Design review of the part built by this model. Coordinates are the model's own, in mm. A direction names the side the tool comes from. Give positions to 0.01 mm unless a question says otherwise; leave off trailing zeros. Write each loop counter-clockwise with the first axis right and the second up, starting at its lowest first coordinate (ties: lowest second). Pieces come first, ordered by that corner, then holes. Notation, with made-up numbers: (49.5, 36) -> (100.5, 36) arc R16 cw to (100.5, 57) -> close; hole circle Ø9 at (-23.75, 46). An arc over 180 degrees is marked (long way). Put each result on its own line as item: value. Start each with the question number.
from build123d import *

# Parameters (mm, degrees)
SCHIZZO4_R               = 2
TAGLIO_ESTRUSIONE1_DEPTH = 8


with BuildPart() as part:
    # Schizzo3 → Rivoluzione1 (revolve)
    with BuildSketch(Plane(origin=(0, 0, 0), x_dir=(1, 0, 0), z_dir=(0, 1, 0))):
        Polygon((0, 0), (0, 19.5), (21, 19.5), (21, 18.5), (53.5, 18.5), (53.5, 17.5), (58, 17.5), (58, 20.25), (93, 20.25), (93, 9.75), (98, 9.75), (98, 4), (112, 4), (112, 0), align=None)
    revolve(axis=Axis((112, 0, 0), (-1, 0, 0)))

    # Schizzo4 → Taglio-Estrusione1 (cut)
    with BuildSketch(Plane(origin=(93, 0, 0), x_dir=(0, 0, -1), z_dir=(1, 0, 0))):
        with Locations((0, 15)):
            Circle(SCHIZZO4_R)
        with Locations((12.990381057, -7.5)):
            Circle(SCHIZZO4_R)
        with Locations((-12.990381057, -7.5)):
            Circle(SCHIZZO4_R)
    extrude(amount=-TAGLIO_ESTRUSIONE1_DEPTH, mode=Mode.SUBTRACT)


solid = part.part
Q1. Take a section at D-D on z = -12. Give the boundary of the cut face in (x, y).
Q2. For pin 1 (1.2 mm diameter, centred on y = -7.5, z = 13, fed in from +X); pin 2 (6 mm diameter, centred on x = 33.5, z = 15, fed in from +Y); pin 3 (1 mm diameter, centred on x = 30.5, y = 1.5, fed in from +Z), all flat-tipped, find the tip position at first contact; note any pin that passes through.
Q3. Mouldability with a two-part tool opening along X and no side actions: class faces 1 (the face through (21, 7.13, -17.24)), 2 (the face through (98, -0.1, -4.2)), 3 (the face through (0, 0, 0)), 4 (the face through (89.056, -6.148, -11.516)) as +X half, -X half, draft (parallel to the pull), parting line (faces both ways), or undercut.
Q4. Machinability: for faces 5 (the face through (10.647, -19.334, 2.539)), 6 (the face through (76, -17, -11)), 7 (the face through (85, -7, -13)), 8 (the face through (58, 6, -17)), which of the approach directions +Z, -Z, +X, -X, +Y, -Y give a long, thin tool a straight path to every point of the face, cutting with its end or side? Answer none if there is none.
Q5. Take a section at C-C on x = 102.5. Give the boundary of the cut face in (y, z).
Q6. To check wall thickness, follow probe 1 along Y at (x, z) = (90.75, 0); probe 2 along X at (y, z) = (-14, 13); probe 3 along Z at (x, y) = (65.5, 5.5). State the ranges of each line that lie inside material, in increasing order. Write a range as from..to.
Q7. Take a section at B-B on y = 0. Give the boundary of the cut face in (x, z), then the cut area to 3 significant figures.
Q8. Take a section at A-A on z = 0. Give the boundary of the cut face in (x, y), then the cut area to 3 significant figures.
Result:
1. outline: (0, -15.37) -> (21, -15.37) -> (21, -14.08) -> (53.5, -14.08) -> (53.5, -12.74) -> (58, -12.74) -> (58, -16.31) -> (93, -16.31) -> (93, -9.24) -> (85, -9.24) -> (85, -5.76) -> (93, -5.76) -> (93, 16.31) -> (58, 16.31) -> (58, 12.74) -> (53.5, 12.74) -> (53.5, 14.08) -> (21, 14.08) -> (21, 15.37) -> (0, 15.37) -> close
2. pin 1: stops at x = 85
2. pin 2: stops at y = 14.08
2. pin 3: stops at z = 18.47
3. face 1: undercut
3. face 2: +X half
3. face 3: -X half
3. face 4: draft
4. face 5: -X
4. face 6: +X, -X
4. face 7: +X
4. face 8: none
5. outline: circle Ø8 at (0, 0)
6. probe 1: y = -20.25..13, 17..20.25
6. probe 2: x = 0..21, 58..93
6. probe 3: z = -19.49..19.49
7. outline: (0, -19.5) -> (21, -19.5) -> (21, -18.5) -> (53.5, -18.5) -> (53.5, -17.5) -> (58, -17.5) -> (58, -20.25) -> (93, -20.25) -> (93, -9.75) -> (98, -9.75) -> (98, -4) -> (112, -4) -> (112, 4) -> (98, 4) -> (98, 9.75) -> (93, 9.75) -> (93, 20.25) -> (58, 20.25) -> (58, 17.5) -> (53.5, 17.5) -> (53.5, 18.5) -> (21, 18.5) -> (21, 19.5) -> (0, 19.5) -> close
7. area: 3,810 mm^2
8. outline: (0, -19.5) -> (21, -19.5) -> (21, -18.5) -> (53.5, -18.5) -> (53.5, -17.5) -> (58, -17.5) -> (58, -20.25) -> (93, -20.25) -> (93, -9.75) -> (98, -9.75) -> (98, -4) -> (112, -4) -> (112, 4) -> (98, 4) -> (98, 9.75) -> (93, 9.75) -> (93, 13) -> (85, 13) -> (85, 17) -> (93, 17) -> (93, 20.25) -> (58, 20.25) -> (58, 17.5) -> (53.5, 17.5) -> (53.5, 18.5) -> (21, 18.5) -> (21, 19.5) -> (0, 19.5) -> close
8. area: 3,770 mm^2
